Verification items for this drawing (mm, ordinates from the low corner). A direction names the side the tool comes from. Give positions to 0.01 mm unless a question says otherwise; leave off trailing zeros. Order: outer loops, then holes, each group sorted by start corner. A loop starts at its lowest first (then second) coordinate and runs counter-clockwise, first axis right, second up. Notation, with made-up numbers: M 58.25,80 L 108.25,80 A11 cw 108.25,96 Z; hole C 82,55 d3. An arc over 180 degrees is marked long. Answer as a JSON object with one key per item and string values.
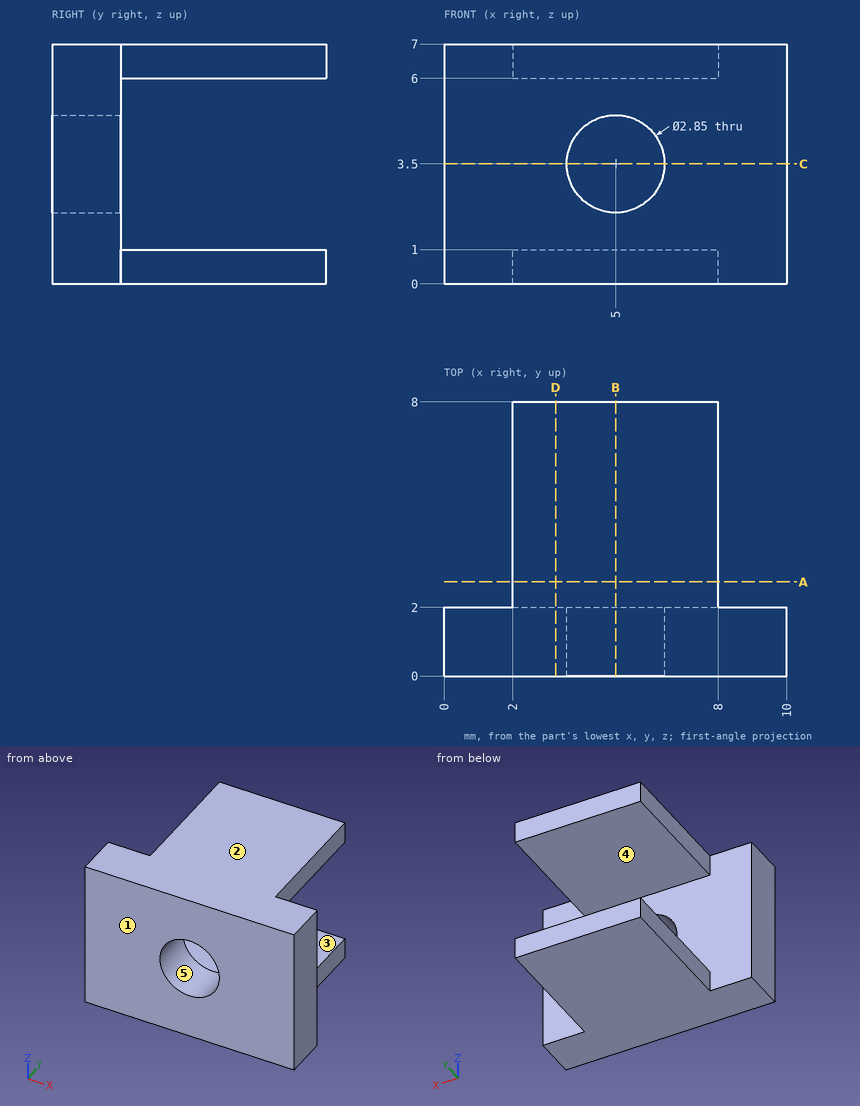
Q1. Material ranges on L1, parallel to X at y = 1.55, z = 3.5 (3 decimals); L2, parallel to Z at x = 5, y = 1.3 (3 decimals); L3, parallel to Z at x = 5, y = 6.5, recorded low to high.
Resolved:
{"L1": "x = 0 to 3.575, 6.425 to 10", "L2": "z = 0 to 2.075, 4.925 to 7", "L3": "z = 0 to 1, 6 to 7"}
Q2. Section check A-A on y = 2.75. Record the cut outline in (x, z).
Resolved:
{"outline": "M 2,0 L 8,0 L 8,1 L 2,1 Z; M 2,6 L 8,6 L 8,7 L 2,7 Z"}
Q3. Release check for a two-part mould opening along Z. For the marked faces 1, 2 and 3 record: +Z half, -Z half, draft (parallel to the pull), parting line (faces both ways), or undercut.
Resolved:
{"face 1": "draft", "face 2": "+Z half", "face 3": "undercut"}
Q4. Section check C-C on z = 3.5. Record the cut outline in (x, y) (3 decimals), then the cut area to 3 significant figures.
Resolved:
{"outline": "M 0,0 L 3.575,0 L 3.575,2 L 0,2 Z; M 6.425,0 L 10,0 L 10,2 L 6.425,2 Z", "area": "14.3 mm²"}
Q5. Gauge pin test, flat ends, axial feed: pin 1 Ø0.8 at (y, z) = (6.5, 6.5) entering from -X; pin 2 Ø0.8 at (y, z) = (6, 0.5) entering from +X; pin 3 Ø2.5 at (x, z) = (5, 3.5) entering from +Y. Record the tip position at first contact, or that the pin passes through.
Resolved:
{"pin 1": "stops at x = 2", "pin 2": "stops at x = 8", "pin 3": "passes through"}
Q6. Tool access check on the marked faces 4 and 5. Record the directions out of +Z, -Z, +X, -X, +Y, -Y that give a thin tool (end or side, any length) a straight path to the whole face; none if there is none.
Resolved:
{"face 4": "+X, -X, +Y", "face 5": "+Y, -Y"}
Q7. Section check D-D on x = 3.25. Record the cut outline in (y, z), then the cut area to 3 significant figures.
Resolved:
{"outline": "M 0,0 L 8,0 L 8,1 L 2,1 L 2,6 L 8,6 L 8,7 L 0,7 Z", "area": "26.0 mm²"}
Q8. Section check B-B on x = 5. Record the cut outline in (y, z) (3 decimals).
Resolved:
{"outline": "M 0,0 L 8,0 L 8,1 L 2,1 L 2,2.075 L 0,2.075 Z; M 0,4.925 L 2,4.925 L 2,6 L 8,6 L 8,7 L 0,7 Z"}
